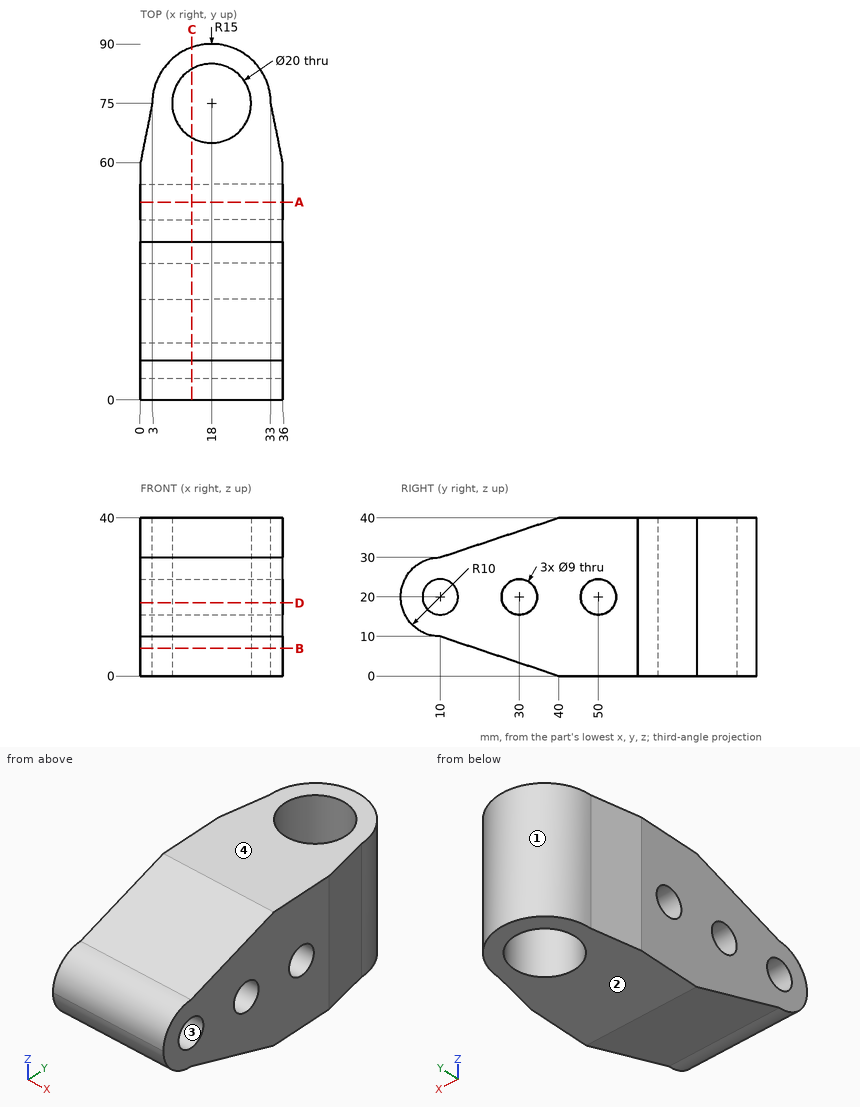
Geometry: see drawing. Coordinates: mm, zero at the bounding-box minimum. Coordinates: 2 decimals unless noted, no trailing zeros. Loops run counter-clockwise (first coordinate to the right, second up) from the corner with the lowest first, then second, coordinate; pieces in that order, holes last. Notation, with made-up numbers: (-35.75, -24.5) - (-4.75, -24.5) arc R28 ccw to (-4.75, -5.5) - close; hole circle Ø7 at (0.25, 56.25). An arc over 180 degrees is marked (long way). Put each result on its own line as item: value. Start each with the question number.
Q1. Cut plane C-C, the plane x = 13. Return loops of the section in (y, z), and give its area (3 significant figures).
Q2. Pin query (flat end, axial travel): pin 1 Ø14.5 at (y, z) = (50, 20) entering from -X; pin 2 Ø5 at (x, y) = (20, 14) entering from -Z; pin 3 Ø5.5 at (y, z) = (10, 20) entering from +X; pin 4 Ø10 at (x, y) = (13.5, 26.5) entering from -Z. Return the tip coordinate at first contact, or that it passes through.
Q3. Pull-direction query (Z, two-part tool) for the marked faces 1, 2, 3 and 4; classes: released by +Z, released by -Z, zero draft, split by the parting line, or undercut.
Q4. Cut plane B-B, the plane z = 7. Return loops of the section in (x, y).
Q5. Cut plane D-D, the plane z = 18.5. Return loops of the section in (x, y).
Q6. Line query: line 1 (Y direction, x = 11.25, z = 20); line 2 (Y direction, x = 24, z = 20); line 3 (X direction, y = 75.5, z = 4.5). Output: solid intervals per line, ascending.
Q7. Cut plane A-A, the plane y = 50. Return loops of the section in (x, z).
Filled sheet:
1. outline: (10, 10) - (40, 0) - (66.34, 0) - (66.34, 40) - (40, 40) - (10, 30) arc R10 ccw to start; (83.66, 0) - (89.14, 0) - (89.14, 40) - (83.66, 40) - close; hole circle Ø9 at (10, 20); hole circle Ø9 at (30, 20); hole circle Ø9 at (50, 20)
1. area: 2,140 mm²
2. pin 1: x = 0
2. pin 2: z = 7.83
2. pin 3: through
2. pin 4: z = 2.83
3. face 1: zero draft
3. face 2: released by -Z
3. face 3: undercut
3. face 4: released by +Z
4. outline: (0, 19) - (36, 19) - (36, 60) - (33, 75) arc R15 ccw to (3, 75) - (0, 60) - close; hole circle Ø20 at (18, 75)
5. outline: (0, 0.11) - (36, 0.11) - (36, 5.76) - (0, 5.76) - close; (0, 14.24) - (36, 14.24) - (36, 25.76) - (0, 25.76) - close; (0, 34.24) - (36, 34.24) - (36, 45.76) - (0, 45.76) - close; (0, 54.24) - (36, 54.24) - (36, 60) - (33, 75) arc R15 ccw to (3, 75) - (0, 60) - close; hole circle Ø20 at (18, 75)
6. line 1: 0 to 5.5, 14.5 to 25.5, 34.5 to 45.5, 54.5 to 67.62, 82.38 to 88.4
6. line 2: 0 to 5.5, 14.5 to 25.5, 34.5 to 45.5, 54.5 to 67, 83 to 88.75
6. line 3: 3.01 to 8.01, 27.99 to 32.99
7. outline: (0, 0) - (36, 0) - (36, 15.5) - (0, 15.5) - close; (0, 24.5) - (36, 24.5) - (36, 40) - (0, 40) - close
